from build123d import *

# Parameters (mm, degrees)
BOSS_EXTRUDE1_DEPTH = 170.165700006
FILLET1_R           = 0.508
FILLET2_R           = 2.794


with BuildPart() as part:
    # Sketch1 → Boss-Extrude1 (new body)
    with BuildSketch(Plane(origin=(0, 0, 0), x_dir=(0, 0, -1), z_dir=(1, 0, 0))):
        Polygon((0.09779276, -0.0508), (14.70220724, -0.0508), (10.623611135, -5.8542), (4.176388865, -5.8542), align=None)
    extrude(amount=BOSS_EXTRUDE1_DEPTH)

    # Fillet1
    fillet1_edges = [part.edges().sort_by_distance(p)[0] for p in [
        (85.082850003, -0.0508, -0.09779276),
        (85.082850003, -0.0508, -14.70220724),
    ]]
    fillet(fillet1_edges, radius=FILLET1_R)

    # Fillet2
    fillet2_edges = [part.edges().sort_by_distance(p)[0] for p in [
        (85.082850003, -5.8542, -10.623611135),
        (85.082850003, -5.8542, -4.176388865),
    ]]
    fillet(fillet2_edges, radius=FILLET2_R)


solid = part.part
Read the model definition and answer for the solid it produces. Units are mm, in the model's axes. Coordinates: 2 decimals unless noted, no trailing zeros. Loops run counter-clockwise (first coordinate to the right, second up) from the corner with the lowest first, then second, coordinate; pieces in that order, holes last.
Q1. The part is cut by section A-A on x = 89. Write down the section's boundary in (y, z).
Q2. Consider probe 1 along Y at (x, z) = (12.5, -9.25); probe 2 along Z at (x, y) = (7.5, -4.7); probe 3 along Z at (x, y) = (67.5, -0.4). Determine where each line is inside the solid, lowest interval first.
Q3. Each of these flat-tipped pins is pushed along its axis until it touches: pin 1 Ø2 at (x, y) = (46.5, -2.5) entering from -Z; pin 2 Ø1.5 at (x, z) = (148, -5) entering from -Y. Where does it stop, or does it pass through?
Q4. The part is cut by section B-B on y = -3.1. Write down the section's boundary in (x, z).
Results below:
1. outline: (-5.85, -9.17) arc R2.79 ccw to (-4.67, -11.46) - (-0.85, -14.14) arc R0.51 ccw to (-0.05, -13.72) - (-0.05, -1.08) arc R0.51 ccw to (-0.85, -0.66) - (-4.67, -3.34) arc R2.79 ccw to (-5.85, -5.63) - close
2. probe 1: y = -5.85 to -0.05
2. probe 2: z = -11.43 to -3.37
2. probe 3: z = -14.21 to -0.59
3. pin 1: stops at z = -13.68
3. pin 2: stops at y = -5.85
4. outline: (0, -12.56) - (170.17, -12.56) - (170.17, -2.24) - (0, -2.24) - close
